Check sheet for the modelled part. Datum: model origin and axes. Units: mm. Face numbers are marked on the shaded views. A direction names the side the tool comes from. Give positions to 0.01 mm unless a question says otherwise; leave off trailing zeros. Write each loop counter-clockwise with the first axis right and the second up, starting at its lowest first coordinate (ties: lowest second). Pieces come first, ordered by that corner, then holes. Notation, with made-up numbers: (86.5, 67) -> (129.5, 67) arc R19 cw to (129.5, 88) -> close; hole circle Ø6 at (32, 8.5). An arc over 180 degrees is marked (long way). Answer as a JSON object with one key per item and string values.
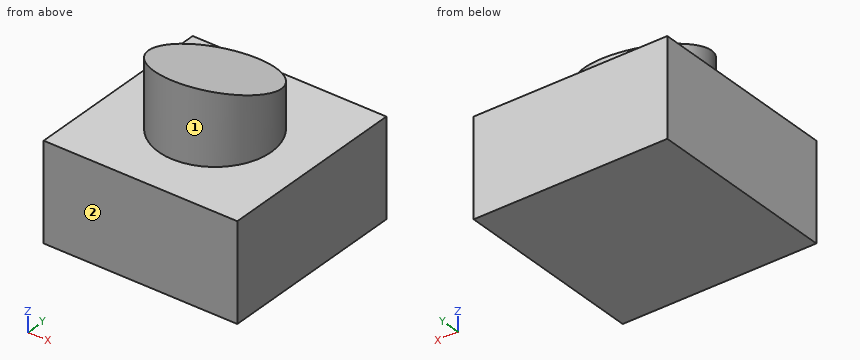
from build123d import *

# Parameters (mm, degrees)
F0_W     = 50.8
F0_H     = 50.8
F1_DEPTH = 25.4
F2_R     = 14.772964705
F3_DEPTH = 25.4
F5_DEPTH = 25.4


with BuildPart() as f1:
    # F0 (on Top) → F1 (new body)
    with BuildSketch(Plane.XY):
        Rectangle(F0_W, F0_H)
    extrude(amount=-F1_DEPTH)

    # F2 (on face) → F3 (join)
    with BuildSketch(Plane.XY):
        Circle(F2_R)
    extrude(amount=F3_DEPTH)

    # F4 (on Right) → F5 (cut, symmetric)
    with BuildSketch(Plane.YZ):
        Polygon((-22.9588039219, 40.4620580375), (-20.6856597215, 21.3676057756), (29.3236263096, 5.0009298138), (29.3236263096, 40.4620580375), align=None)
    extrude(amount=F5_DEPTH, both=True, mode=Mode.SUBTRACT)


solid = f1.part
1. Go/stop test with flat-tipped pins: P1, Ø2, axis at x = 16, z = 4, coming from the +Y side; P2, Ø1, axis at x = -10, y = 4, coming from the +Z side; P3, Ø10, axis at y = 12.5, z = 6, coming from the +X side. Record where each tip stops, or that it passes through.
Determined:
{"P1": "through", "P2": "z = 13.45", "P3": "x = 12.73"}
2. Sectioned sample at B-B, the plane z = 9. Enter the section's corners in (x, y).
Determined:
{"outline": "circle Ø29.55 at (0, 0)"}
3. Scan lines: L1, parallel to Z at x = -12.5, y = -8; L2, parallel to Y at x = -5, z = 2; L3, parallel to X at y = -10, z = 10. Record each from-to range of solid material in increasing order. Write a range as [from, to].
Determined:
{"L1": "[-25.4, 0]", "L2": "[-13.9, 13.9]", "L3": "[-10.87, 10.87]"}
4. Sectioned sample at C-C, the plane y = 5.5. Enter the section's corners in (x, z).
Determined:
{"outline": "(-25.4, -25.4) -> (25.4, -25.4) -> (25.4, 0) -> (13.71, 0) -> (13.71, 12.8) -> (-13.71, 12.8) -> (-13.71, 0) -> (-25.4, 0) -> close"}
5. Access from +Z, -Z, +X, -X, +Y, -Y to the whole of each face (thin tool, end or side, straight path). Record for the marked faces 1 and 2.
Determined:
{"face 1": "+Z", "face 2": "+Z, -Z, +X, -X, -Y"}
6. Sectioned sample at D-D, the plane y = 19. Enter the section's corners in (x, z), plus the area to 3 significant figures.
Determined:
{"outline": "(-25.4, -25.4) -> (25.4, -25.4) -> (25.4, 0) -> (-25.4, 0) -> close", "area": "1,290 mm^2"}
7. Sectioned sample at A-A, the plane x = 0. Enter the section's corners in (y, z), plus the area to 3 significant figures.
Determined:
{"outline": "(-25.4, -25.4) -> (25.4, -25.4) -> (25.4, 0) -> (14.77, 0) -> (14.77, 9.76) -> (-14.77, 19.43) -> (-14.77, 0) -> (-25.4, 0) -> close", "area": "1,720 mm^2"}
